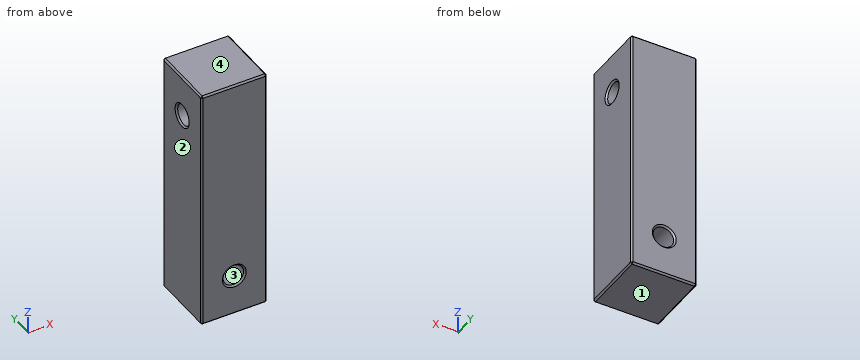
from build123d import *

# Parameters (mm, degrees)
SKETCH_1_W         = 8
SKETCH_1_H         = 8
EXTRUDE_1_DEPTH    = 15
HOLE_WIZARD_M3_1_D = 2.5
HOLE_WIZARD_M3_2_D = 2.5
CHAMFER_1_SIZE     = 0.2


with BuildPart() as part:
    # 草图1 → 凸台-拉伸1 (new, symmetric)
    with BuildSketch(Plane.XY):
        Rectangle(SKETCH_1_W, SKETCH_1_H)
    extrude(amount=EXTRUDE_1_DEPTH, both=True)

    # M3 螺纹孔1 (through all)
    with Locations(Plane(origin=(4, 0, 0), x_dir=(0, 0, -1), z_dir=(1, 0, 0))):
        with Locations((-10, 0)):
            Hole(HOLE_WIZARD_M3_1_D / 2)

    # M3 螺纹孔2 (through all)
    with Locations(Plane(origin=(0, 4, 0), x_dir=(1, 0, 0), z_dir=(0, 1, 0))):
        with Locations((0, 10)):
            Hole(HOLE_WIZARD_M3_2_D / 2)

    # 倒角1
    chamfer_1_edges = [part.edges().sort_by_distance(p)[0] for p in [
        (-4, 0, 15),
        (4, 0, 8.75),
        (-4, 0, 8.75),
        (0, -4, 15),
        (1.25, 4, -10),
        (1.25, -4, -10),
        (4, 0, 15),
        (0, -4, -15),
        (-4, 0, -15),
        (0, 4, -15),
        (4, 0, -15),
        (4, -4, 0),
        (-4, -4, 0),
        (-4, 4, 0),
        (4, 4, 0),
        (0, 4, 15),
    ]]
    chamfer(chamfer_1_edges, length=CHAMFER_1_SIZE)


solid = part.part
Could you check a few things on this model? Use its own coordinates, in mm. Face numbers are marked on the shaded views. Round coordinates to 2 decimals unless told otherwise and drop trailing zeros. Write each loop counter-clockwise with the first axis right and the second up, starting at its lowest first coordinate (ties: lowest second). Pieces come first, ordered by that corner, then holes. Notation, with made-up numbers: (34, -2) - (69, -2) arc R26 cw to (69, 30) - close; hole circle Ø11 at (-7.75, 17). An arc over 180 degrees is marked (long way). Put each result on its own line as item: value. Start each with the question number.
(1) Thinking about a two-plate mould opening in Z: for the marked faces 1, 2, 3 and 4, which applies, released by +Z, released by -Z, zero draft, split by the parting line, or undercut?
(2) I want a section at A-A, the plane x = 0. Please give me the cut outline in (y, z), plus the area to 3 significant figures.
(3) I want a section at B-B, the plane z = -10. Please give me the cut outline in (x, y).
(4) I want a section at C-C, the plane x = 2.5. Please give me the cut outline in (y, z), plus the area to 3 significant figures.
(5) I need wall thicknesses on probe 1 along X at (y, z) = (1.75, -10); probe 2 along Z at (x, y) = (0, 0.5). Which ranges of each line are inside material? Lowest first, please.
Here are the results:
1. face 1: released by -Z
1. face 2: zero draft
1. face 3: undercut
1. face 4: released by +Z
2. outline: (-4, -14.8) - (-3.8, -15) - (3.8, -15) - (4, -14.8) - (4, -11.45) - (3.8, -11.25) - (-3.8, -11.25) - (-4, -11.45) - close; (-4, -8.55) - (-3.8, -8.75) - (3.8, -8.75) - (4, -8.55) - (4, 14.8) - (3.8, 15) - (-3.8, 15) - (-4, 14.8) - close; hole circle Ø2.5 at (0, 10)
2. area: 215 mm^2
3. outline: (-4, -3.8) - (-3.8, -4) - (-1.45, -4) - (-1.25, -3.8) - (-1.25, 3.8) - (-1.45, 4) - (-3.8, 4) - (-4, 3.8) - close; (1.25, -3.8) - (1.45, -4) - (3.8, -4) - (4, -3.8) - (4, 3.8) - (3.8, 4) - (1.45, 4) - (1.25, 3.8) - close
4. outline: (-4, -14.8) - (-3.8, -15) - (3.8, -15) - (4, -14.8) - (4, 14.8) - (3.8, 15) - (-3.8, 15) - (-4, 14.8) - close; hole circle Ø2.5 at (0, 10)
4. area: 235 mm^2
5. probe 1: x = -4 to -1.25, 1.25 to 4
5. probe 2: z = -15 to -11.25, -8.75 to 8.85, 11.15 to 15
